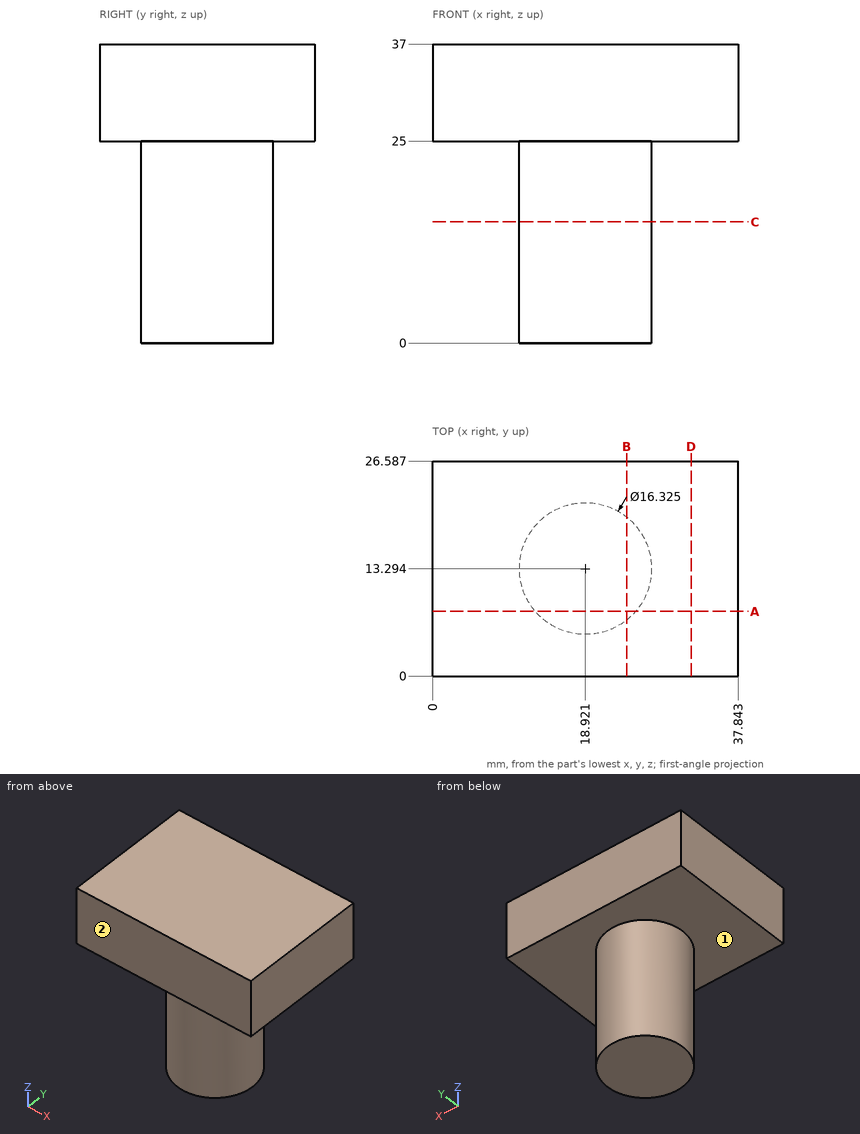
Here's the drawing with two shaded views (mm, measured from the low corner). I have some questions. A direction names the side the tool comes from. Give positions to 0.01 mm unless a question says otherwise; leave off trailing zeros. Loops run counter-clockwise (first coordinate to the right, second up) from the corner with the lowest first, then second, coordinate; pieces in that order, holes last. Notation, with made-up numbers: M 1.5,55.5 L 12.5,55.5 A33 cw 12.5,84.5 Z; hole C 51.5,0.25 d9. An arc over 180 degrees is marked long. One line per item, written item: value. Start each with the question number.
1) If I drill on line 1 (Z direction, x = 33.5, y = 8.5); line 2 (X direction, y = 18.5, z = 6.5) (1 decimal); line 3 (Y direction, x = 12.5, z = 5.5) (1 decimal), over which ranges is the centre line in solid material (lowest first)? Write a range as [from, to].
2) I'm going to push flat-ended pins straight in: pin 1 (1.5 mm diameter, centred on x = 14.5, y = 9.5, fed in from -Z); pin 2 (6 mm diameter, centred on x = 29, y = 5, fed in from -Z); pin 3 (8 mm diameter, centred on x = 11, z = 13, fed in from -Y) (1 decimal); pin 4 (1.5 mm diameter, centred on y = 18.5, z = 9, fed in from -X). Where does each tip first touch, or does it pass through?
3) If we section it at B-B, the plane x = 24: Write out the boundary of the cut face in (y, z).
4) On a 3-axis mill with a long thin cutter (end or side, diameter ignored), from which of +Z, -Z, +X, -X, +Y, -Y can I reach the whole of each face in a straight line? I mean the marked faces 1 and 2. Say none if no direction works.
5) If we section it at C-C, the plane z = 15: Write out the boundary of the cut face in (x, y) (1 decimal), and give its area (3 significant figures).
6) If we section it at D-D, the plane x = 32: Write out the boundary of the cut face in (y, z).
7) If we section it at A-A, the plane y = 8: Write out the boundary of the cut face in (x, z) (1 decimal).
Completed:
1. line 1: z = [25, 37]
1. line 2: x = [12.6, 25.2]
1. line 3: y = [8.3, 18.3]
2. pin 1: stops at z = 0
2. pin 2: stops at z = 25
2. pin 3: stops at y = 6.1
2. pin 4: stops at x = 12.08
3. outline: M 0,25 L 6.9,25 L 6.9,0 L 19.68,0 L 19.68,25 L 26.59,25 L 26.59,37 L 0,37 Z
4. face 1: -Z
4. face 2: +Z, -Z, +X, -X, -Y
5. outline: C 18.9,13.3 d16.3
5. area: 209 mm^2
6. outline: M 0,25 L 26.59,25 L 26.59,37 L 0,37 Z
7. outline: M 0,25 L 12.7,25 L 12.7,0 L 25.1,0 L 25.1,25 L 37.8,25 L 37.8,37 L 0,37 Z
